Source: CAD feature listing. Evaluate the final solid. Frame: model axes, mm. Face numbers are marked on the shaded views. A direction names the side the tool comes from. Give positions to 0.01 mm unless a question says otherwise; leave off trailing zeros. Loops run counter-clockwise (first coordinate to the right, second up) from the corner with the lowest first, then second, coordinate; pieces in that order, holes last. Notation, with made-up numbers: (84.5, 25) -> (117.5, 25) arc R8 ccw to (117.5, 36) -> close; hole circle Ø5 at (84, -8). An arc over 180 degrees is marked (long way). Put each result on its own line as item: value.
Autodesk Fusion 360 part; units mm, degrees
sketch "Sketch1" plane through (0, 0, 0) normal (0, 0, 1) x (1, 0, 0)
  line L0 (0, 0) -> (20, 0)
  line L1 (20, 0) -> (20, 20)
  line L2 (20, 20) -> (0, 20)
  line L3 (0, 20) -> (0, 0)
  line L4 (0, 0) -> (3, 0)
  line L5 (3, 0) -> (3, 20)
  line L6 (3, 20) -> (0, 20)
  line L7 (0, 20) -> (0, 0)
  line L8 (10, 0) -> (10, 20) construction
  circle A0 centre (10, 10) radius 2.5
  dimension "d7" = 20
  dimension "d8" = 20
  dimension "d9" = 3
  dimension "d10" = 20
  dimension "d12" = 5
extrude "Extrude1" add sketch "Sketch1" along normal blind 3
extrude "Extrude2" add sketch "Sketch1" along normal blind 38 contours L0 L2 L3 L4 L5 L6 L7
sketch "Sketch2" plane through (0, 0, 0) normal (-1, 0, 0) x (0, -1, 0)
  line L0 (-20, 0) -> (0, 0)
  line L1 (0, 0) -> (0, 38)
  line L2 (0, 38) -> (-20, 38)
  line L3 (-20, 38) -> (-20, 0)
  line L4 (-20, 38) -> (0, 18) construction
  line L5 (-20, 38) -> (8.2843, 38) construction
  line L6 (-10, 38) -> (-10, 0) construction
  circle A0 centre (-10, 28) radius 3.5
  dimension "d17" = 45
  dimension "d18" = 7
extrude "Extrude3" cut sketch "Sketch2" against normal up to surface (3 mm away) contours A0
sketch "Sketch3" plane through (3, 0, 0) normal (1, 0, 0) x (0, 1, 0)
  circle A0 centre (10, 28) radius 3.5
  line L0 (0, 3) -> (20, 3)
  line L1 (20, 3) -> (20, 38)
  line L2 (20, 38) -> (0, 38)
  line L3 (0, 38) -> (0, 3)
  line L4 (10, 28) -> (10, 29.25)
  line L5 (10, 29.25) -> (19, 29.25)
  line L6 (19, 29.25) -> (19, 26.75)
  line L7 (19, 26.75) -> (10, 26.75)
  line L8 (10, 26.75) -> (10, 29.25)
  dimension "d21" = 1.25
  dimension "d23" = 9
  dimension "d24" = 2.5
extrude "Extrude4" cut sketch "Sketch3" against normal blind 2.5 contours A0 L5 L6 L7
equation "pot_hole_diameter = 7 mm"
equation "pot_turn_stop_slot_depth = 2.5 mm"
equation "pot_turn_stop_slot_width = 2.5 mm"
equation "thickness = 3 mm"
equation "mount_width = 20 mm"
equation "mount_height = 35 mm"
equation "d7 = mount_width"
equation "d8 = mount_width"
equation "d9 = thickness"
equation "d10 = mount_width"
equation "screw_hole_diameter = 5 mm"
equation "d12 = screw_hole_diameter"
equation "d13 = thickness"
equation "d15 = thickness + mount_height"
equation "d18 = pot_hole_diameter"
equation "d21 = pot_turn_stop_slot_width / 2"
equation "pot_slot_length = 9 mm"
equation "d23 = pot_slot_length"
equation "d24 = pot_turn_stop_slot_width"
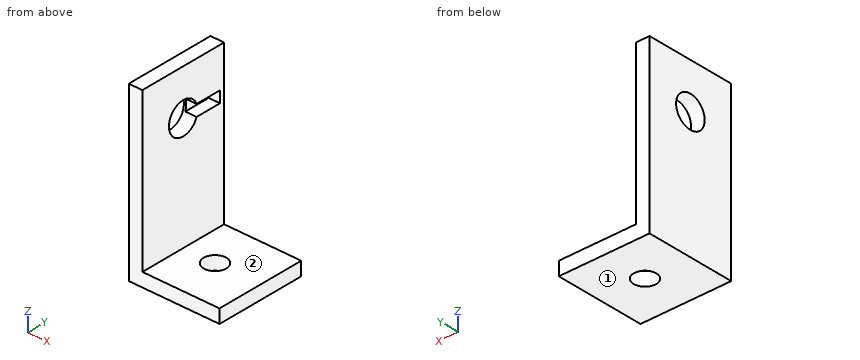
(1) Section A-A on x = 10. Return loops of the section in (y, z), then the cut area to 3 significant figures.
Calculated:
outline: (0, 0) -> (7.5, 0) -> (7.5, 3) -> (0, 3) -> close; (12.5, 0) -> (20, 0) -> (20, 3) -> (12.5, 3) -> close
area: 45.0 mm²
(2) Line query: probe 1 along Y at (x, z) = (1.15, 28); probe 2 along Z at (x, y) = (0.8, 10); probe 3 along Y at (x, z) = (10, 1). Output: solid intervals per line, ascending. Write a range as from..to.
Calculated:
probe 1: y = 0..6.5, 19..20
probe 2: z = 0..24.5, 31.5..38
probe 3: y = 0..7.5, 12.5..20
(3) First-contact query: P1, Ø0.8, axis at x = 1, y = 17.5, coming from the -Z side; P2, Ø6, axis at y = 3.5, z = 25.5, coming from the +X side; P3, Ø6, axis at x = 7.5, z = 10, coming from the -Y side; P4, Ø0.8, axis at y = 17.5, z = 28.5, coming from the +X side. Flat tips, straight axial feed; report the tip coordinate or a pass-through.
Calculated:
P1: stops at z = 0
P2: stops at x = 3
P3: passes through
P4: stops at x = 0.5
(4) Section B-B on y = 10. Return loops of the section in (x, z), then the cut area to 3 significant figures.
Calculated:
outline: (0, 0) -> (7.5, 0) -> (7.5, 3) -> (3, 3) -> (3, 24.5) -> (0, 24.5) -> close; (0, 31.5) -> (3, 31.5) -> (3, 38) -> (0, 38) -> close; (12.5, 0) -> (20, 0) -> (20, 3) -> (12.5, 3) -> close
area: 129 mm²
(5) Section C-C on z = 28. Return loops of the section in (x, y).
Calculated:
outline: (0, 0) -> (3, 0) -> (3, 6.5) -> (0, 6.5) -> close; (0, 13.5) -> (0.5, 13.5) -> (0.5, 19) -> (3, 19) -> (3, 20) -> (0, 20) -> close
(6) Section D-D on y = 5. Return loops of the section in (x, z), then the cut area to 3 significant figures.
Calculated:
outline: (0, 0) -> (20, 0) -> (20, 3) -> (3, 3) -> (3, 38) -> (0, 38) -> close
area: 165 mm²
(7) Reachability of the marked faces 1 and 2 from +Z, -Z, +X, -X, +Y, -Y: full face, straight path, thin tool, end or side. Return the list, or none.
Calculated:
face 1: -Z, +X, -X, +Y, -Y
face 2: +Z, +X, +Y, -Y
